```python
from build123d import *

# Parameters (mm, degrees)
SKETCH2_R                = 25.5
BASE_FLANGE1_DEPTH       = 1.21
M2_CLEARANCE_HOLE1_D     = 2.4
M2_CLEARANCE_HOLE1_DEPTH = 10
M2_CLEARANCE_HOLE1_TIP   = 0.721032743


# Sheet-metal steps are written as plain solids
with BuildPart() as part:
    # Sketch2 → Base-Flange1 (new body)
    with BuildSketch(Plane(origin=(0, 0, 0), x_dir=(1, 0, 0), z_dir=(0, 1, 0))):
        with Locations(Location((0, 0, 0), (0, 0, 270))):
            Circle(SKETCH2_R)
    extrude(amount=-BASE_FLANGE1_DEPTH)

    # M2 Clearance Hole1
    with Locations(Plane(origin=(0, -1.21, 0), x_dir=(-1, 0, 0), z_dir=(0, -1, 0))):
        with Locations((0, -12.75), (-12.75, 0), (12.75, 0), (0, 12.75)):
            Hole(M2_CLEARANCE_HOLE1_D / 2, depth=M2_CLEARANCE_HOLE1_DEPTH)
            with Locations((0, 0, -(M2_CLEARANCE_HOLE1_DEPTH + M2_CLEARANCE_HOLE1_TIP / 2))):  # 118° drill point
                Cone(0, M2_CLEARANCE_HOLE1_D / 2, M2_CLEARANCE_HOLE1_TIP, mode=Mode.SUBTRACT)


solid = part.part
```
Work out the finished part from the listing and answer in its coordinate system (mm). Give positions to 0.01 mm unless a question says otherwise; leave off trailing zeros. Loops run counter-clockwise (first coordinate to the right, second up) from the corner with the lowest first, then second, coordinate; pieces in that order, holes last. Notation, with made-up numbers: (77, 28.25) -> (96, 28.25) arc R17 ccw to (96, 33.25) -> close; hole circle Ø11 at (-39.75, -7). An arc over 180 degrees is marked (long way). Use CSV: the item, a comma, the result in double quotes.
1. A flat-ended cylindrical pin translates along its axis: pin 1 Ø1.4 at (x, z) = (12.75, 0) entering from -Y. Find the tip coordinate at first contact, or state that the pin passes through.
Found:
pin 1,"through"
2. The part is cut by section A-A (x = 0). Write down the section's boundary in (y, z).
Found:
outline,"(-1.21, -25.5) -> (0, -25.5) -> (0, -13.95) -> (-1.21, -13.95) -> close; (-1.21, -11.55) -> (0, -11.55) -> (0, 11.55) -> (-1.21, 11.55) -> close; (-1.21, 13.95) -> (0, 13.95) -> (0, 25.5) -> (-1.21, 25.5) -> close"
3. The part is cut by section B-B (z = -12.75). Write down the section's boundary in (x, y), then the cut area to 3 significant figures.
Found:
outline,"(-22.08, -1.21) -> (-1.2, -1.21) -> (-1.2, 0) -> (-22.08, 0) -> close; (1.2, -1.21) -> (22.08, -1.21) -> (22.08, 0) -> (1.2, 0) -> close"
area,"50.5 mm^2"
4. Straight lines are drawn through the part: line 1 (X direction, y = -0.45, z = 13); line 2 (Z direction, x = 1, y = -0.75); line 3 (X direction, y = -0.3, z = 18). For each, find the intervals that lie inside material, in ascending order.
Found:
line 1,"-21.94 to -1.17, 1.17 to 21.94"
line 2,"-25.48 to -13.41, -12.09 to 12.09, 13.41 to 25.48"
line 3,"-18.06 to 18.06"
5. The part is cut by section C-C (x = 12.75). Write down the section's boundary in (y, z), then the cut area to 3 significant figures.
Found:
outline,"(-1.21, -22.08) -> (0, -22.08) -> (0, -1.2) -> (-1.21, -1.2) -> close; (-1.21, 1.2) -> (0, 1.2) -> (0, 22.08) -> (-1.21, 22.08) -> close"
area,"50.5 mm^2"
6. The part is cut by section D-D (y = -0.55). Write down the section's boundary in (x, z), then the cut area to 3 significant figures.
Found:
outline,"circle Ø51 at (0, 0); hole circle Ø2.4 at (-12.75, 0); hole circle Ø2.4 at (0, -12.75); hole circle Ø2.4 at (0, 12.75); hole circle Ø2.4 at (12.75, 0)"
area,"2,020 mm^2"
7. The mould has two halves that part along Z. Classify faces 1 (the cylindrical face through (-0.26, -0.6, 13.92)), 2 (the cylindrical face through (-24.9, -0.6, -5.5)), 3 (the flat face through (0, 0, 0)): +Z half, -Z half, draft (parallel to the pull), parting line (faces both ways), or undercut.
Found:
face 1,"undercut"
face 2,"parting line"
face 3,"draft"
